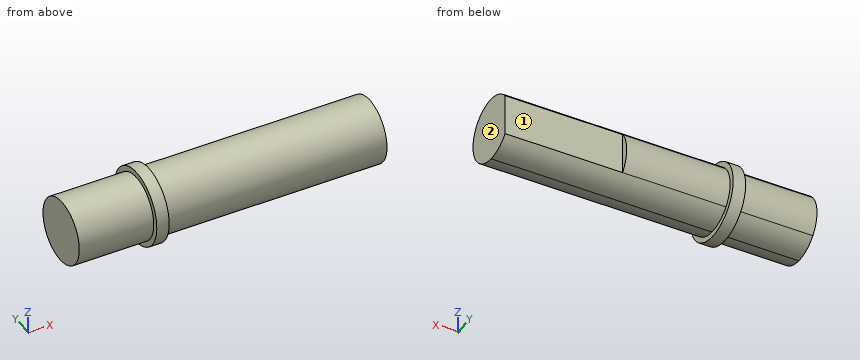
from build123d import *

# Parameters (mm, degrees)
BOSS_EXTRUDE1_DEPTH = 28.2
SKETCH9_6_R         = 4.5
SKETCH9_6_R_2       = 3.85
BOSS_EXTRUDE2_DEPTH = 1.5
BOSS_EXTRUDE3_DEPTH = 14
BOSS_EXTRUDE4_DEPTH = 9


with BuildPart() as part:
    # Sketch9 → Boss-Extrude1 (new body)
    with BuildSketch(Plane(origin=(0, 0, 0), x_dir=(0, 0, -1), z_dir=(1, 0, 0))):
        with BuildLine():
            Line((2.45, 2.969848481), (-2.45, 2.969848481))
            ThreePointArc((-2.45, 2.969848481), (-1.641645516, -3.48245603), (3.85, 0))
            ThreePointArc((3.85, 0), (3.48245603, 1.641645516), (2.45, 2.969848481))
        make_face()
    extrude(amount=BOSS_EXTRUDE1_DEPTH)

    # Sketch9<6> → Boss-Extrude2 (add)
    with BuildSketch(Plane(origin=(0, 0, 0), x_dir=(0, 0, -1), z_dir=(1, 0, 0))):
        Circle(SKETCH9_6_R)
        Circle(SKETCH9_6_R_2, mode=Mode.SUBTRACT)
    extrude(amount=BOSS_EXTRUDE2_DEPTH)

    # Sketch9<7> → Boss-Extrude3 (add)
    with BuildSketch(Plane(origin=(0, 0, 0), x_dir=(0, 0, -1), z_dir=(1, 0, 0))):
        with BuildLine():
            ThreePointArc((2.45, 2.969848481), (0, 3.85), (-2.45, 2.969848481))
            Line((-2.45, 2.969848481), (2.45, 2.969848481))
        make_face()
        with BuildLine():
            Line((2.45, 2.969848481), (-2.45, 2.969848481))
            ThreePointArc((-2.45, 2.969848481), (-1.641645516, -3.48245603), (3.85, 0))
            ThreePointArc((3.85, 0), (3.48245603, 1.641645516), (2.45, 2.969848481))
        make_face()
    extrude(amount=BOSS_EXTRUDE3_DEPTH)

    # Sketch9<8> → Boss-Extrude4 (add)
    with BuildSketch(Plane(origin=(0, 0, 0), x_dir=(0, 0, -1), z_dir=(1, 0, 0))):
        with BuildLine():
            ThreePointArc((2.45, 2.969848481), (0, 3.85), (-2.45, 2.969848481))
            Line((-2.45, 2.969848481), (2.45, 2.969848481))
        make_face()
        with BuildLine():
            Line((2.45, 2.969848481), (-2.45, 2.969848481))
            ThreePointArc((-2.45, 2.969848481), (-1.641645516, -3.48245603), (3.85, 0))
            ThreePointArc((3.85, 0), (3.48245603, 1.641645516), (2.45, 2.969848481))
        make_face()
    extrude(amount=-BOSS_EXTRUDE4_DEPTH)


solid = part.part
Work out the finished part from the listing and answer in its coordinate system (mm). Face numbers are marked on the shaded views. A direction names the side the tool comes from. Give positions to 0.01 mm unless a question says otherwise; leave off trailing zeros. Order: outer loops, then holes, each group sorted by start corner. A loop starts at its lowest first (then second) coordinate and runs counter-clockwise, first axis right, second up. Notation, with made-up numbers: (80, -12) -> (107, -12) arc R25 cw to (107, 22) -> close; hole circle Ø10 at (85, -35.75). An arc over 180 degrees is marked (long way). One line per item, written item: value.
Item 1: Straight lines are drawn through the part: probe 1 along Z at (x, y) = (7.5, 0.25); probe 2 along X at (y, z) = (4, 0.25); probe 3 along Y at (x, z) = (12.5, 0). For each, find the intervals that lie inside material, in ascending order.
Answer sheet:
probe 1: -3.84 to 3.84
probe 2: 0 to 1.5
probe 3: -3.85 to 3.85
Item 2: Find section A-A, the plane y = -3.5. Give the vertices of the cut face in (x, z), plus the area to 3 significant figures.
Answer sheet:
outline: (-9, -1.6) -> (0, -1.6) -> (0, -2.83) -> (1.5, -2.83) -> (1.5, -1.6) -> (28.2, -1.6) -> (28.2, 1.6) -> (1.5, 1.6) -> (1.5, 2.83) -> (0, 2.83) -> (0, 1.6) -> (-9, 1.6) -> close
area: 123 mm²
Item 3: Find section B-B, the plane z = 1.25. Give the vertices of the cut face in (x, y).
Answer sheet:
outline: (-9, -3.64) -> (0, -3.64) -> (0, -4.32) -> (1.5, -4.32) -> (1.5, -3.64) -> (28.2, -3.64) -> (28.2, 2.97) -> (14, 2.97) -> (14, 3.64) -> (1.5, 3.64) -> (1.5, 4.32) -> (0, 4.32) -> (0, 3.64) -> (-9, 3.64) -> close
Item 4: A tool of negligible diameter and unlimited length cuts with its end or side. For the marked faces 1 and 2, from which of +Z, -Z, +X, -X, +Y, -Y can it reach the whole face along a straight path? Write none if from no direction.
Answer sheet:
face 1: +Z, -Z, +X, +Y
face 2: +Z, -Z, +X, +Y, -Y
Item 5: Find section D-D, the plane y = -1. Give the vertices of the cut face in (x, z).
Answer sheet:
outline: (-9, -3.72) -> (0, -3.72) -> (0, -4.39) -> (1.5, -4.39) -> (1.5, -3.72) -> (28.2, -3.72) -> (28.2, 3.72) -> (1.5, 3.72) -> (1.5, 4.39) -> (0, 4.39) -> (0, 3.72) -> (-9, 3.72) -> close
Item 6: Flat-ended cylindrical pins translate along their axes: P1, Ø4, axis at x = 10.5, y = 1.5, coming from the -Z side; P2, Ø2.5, axis at x = 20, z = 0.5, coming from the +Y side; P3, Ø3, axis at x = 18.5, y = -2, coming from the +Z side. Find the tip coordinate at first contact, or state that the pin passes through.
Answer sheet:
P1: z = -3.85
P2: y = 2.97
P3: z = 3.82
Item 7: Find section C-C, the plane x = -5.5. Give the vertices of the cut face in (y, z), plus the area to 3 significant figures.
Answer sheet:
outline: circle Ø7.7 at (0, 0)
area: 46.6 mm²
